Design review of the part built by this model. Coordinates are the model's own, in mm. A direction names the side the tool comes from. Coordinates: 2 decimals unless noted, no trailing zeros. Write each loop counter-clockwise with the first axis right and the second up, starting at its lowest first coordinate (ties: lowest second). Pieces come first, ordered by that corner, then holes. Notation, with made-up numbers: (7, 71.25) - (59, 71.25) arc R19 cw to (59, 89.25) - close; hole circle Ø1 at (36.25, 17). An arc over 180 degrees is marked (long way). One line per item, written item: value.
from build123d import *

# Parameters (mm, degrees)
HIERRO_ANGULAR_1_X_1_X_0_125_1_DEPTH = 200


with BuildPart() as part:
    # Sketch1 → Hierro angular 1 X 1 X 0.125(1) (new body)
    with BuildSketch(Plane.ZX):
        with BuildLine():
            Line((0, 0), (0, 25.4))
            Line((0, 25.4), (0.00508, 25.4))
            ThreePointArc((0.00508, 25.4), (2.246551928, 24.471551928), (3.175, 22.23008))
            Line((3.175, 22.23008), (3.175, 7.9375))
            ThreePointArc((3.175, 7.9375), (4.569903955, 4.569903955), (7.9375, 3.175))
            Line((7.9375, 3.175), (22.23008, 3.175))
            ThreePointArc((22.23008, 3.175), (24.471551928, 2.246551928), (25.4, 0.00508))
            Line((25.4, 0.00508), (25.4, 0))
            Line((25.4, 0), (0, 0))
        make_face()
    extrude(amount=HIERRO_ANGULAR_1_X_1_X_0_125_1_DEPTH)


solid = part.part
1. Consider section C-C, the plane z = 13.5. Write out the cut boundary in (x, y) (3 decimals), then the cut area to 3 significant figures.
Answer block:
outline: (0, 0) - (3.175, 0) - (3.175, 200) - (0, 200) - close
area: 635 mm^2
2. Consider section B-B, the plane x = 17. Write out the cut boundary in (y, z) (3 decimals), then the cut area to 3 significant figures.
Answer block:
outline: (0, 0) - (200, 0) - (200, 3.175) - (0, 3.175) - close
area: 635 mm^2
3. Wall thickness on line 1 along X through (y, z) = (77, 17) (3 decimals); line 2 along X through (y, z) = (98, 6): over which ranges is each line inside the solid? List them lowest first.
Answer block:
line 1: x = 0 to 3.175
line 2: x = 0 to 3.59
4. Insertion check: pin 1 Ø4 at (y, z) = (97.5, 9.5) entering from +X; pin 2 Ø11.5 at (x, y) = (15.5, 65) entering from +Z (3 decimals). Each pin has a flat end and moves straight along its axis. Give the tip position at first contact, or say it passes through.
Answer block:
pin 1: stops at x = 3.2
pin 2: stops at z = 3.175
5. For faces 1 (the face through (0, 99, 13)), 2 (the face through (3.175, 99, 15)), list the 3-axis set-ups (+Z, -Z, +X, -X, +Y, -Y) from which the entire face can be reached by the end or side of a thin tool; tool diameter is ignored.
Answer block:
face 1: +Z, -Z, -X, +Y, -Y
face 2: +Z, +X, +Y, -Y
